```python
from build123d import *

# Parameters (mm, degrees)
SKETCH1_W           = 10
SKETCH1_H           = 10
SKETCH1_R           = 1.5
BOSS_EXTRUDE1_DEPTH = 5
FILLET1_R           = 1.5
SKETCH2_R           = 1.6
BOSS_EXTRUDE2_DEPTH = 1
SKETCH3_R           = 2.25
CUT_EXTRUDE1_DEPTH  = 4


with BuildPart() as part:
    # Sketch1 → Boss-Extrude1 (new body)
    with BuildSketch(Plane.XY):
        with Locations((-140, 155.5)):
            Rectangle(SKETCH1_W, SKETCH1_H)
        with Locations((-140, 155.5)):
            Circle(SKETCH1_R, mode=Mode.SUBTRACT)
    extrude(amount=BOSS_EXTRUDE1_DEPTH)

    # Fillet1
    fillet1_edges = [part.edges().sort_by_distance(p)[0] for p in [
        (-145, 160.5, 2.5),
        (-135, 160.5, 2.5),
        (-135, 150.5, 2.5),
        (-145, 150.5, 2.5),
    ]]
    fillet(fillet1_edges, radius=FILLET1_R)

    # Sketch2 → Boss-Extrude2 (add)
    with BuildSketch(Plane.XY.offset(5)):
        with Locations((-140, 155.5)):
            Circle(SKETCH2_R)
    extrude(amount=-BOSS_EXTRUDE2_DEPTH)

    # Sketch3 → Cut-Extrude1 (cut)
    with BuildSketch(Plane(origin=(0, 0, 0), x_dir=(-1, 0, 0), z_dir=(0, 0, -1))):
        with Locations((140, 155.5)):
            Circle(SKETCH3_R)
    extrude(amount=-CUT_EXTRUDE1_DEPTH, mode=Mode.SUBTRACT)


solid = part.part
```
For this review, take the finished solid that the model builds, in its own axes (mm). A direction names the side the tool comes from. Round coordinates to 2 decimals unless told otherwise and drop trailing zeros. Write each loop counter-clockwise with the first axis right and the second up, starting at its lowest first coordinate (ties: lowest second). Pieces come first, ordered by that corner, then holes. Notation, with made-up numbers: (86.5, 53) - (131.5, 53) arc R19 cw to (131.5, 89) - close; hole circle Ø11 at (32, -33.5). An arc over 180 degrees is marked (long way). Answer as CSV lines item,"result". Start each with the question number.
(1) Add section A-A, the plane y = 155.5. State the section outline as (x, z) points.
(2) Mouldability with a two-part tool opening along Y and no side actions: class faces 3 (the cylindrical face through (-135.45, 150.93, 2.54)), 4 (the flat face through (-140, 158, 0)), 5 (the flat face through (-140, 156, 4)) as +Y half, -Y half, draft (parallel to the pull), parting line (faces both ways), or undercut.
(3) Add section B-B, the plane z = 1.7. State the section outline as (x, y) points, plus the area to 3 significant figures.
(4) Add section D-D, the plane y = 159.5. State the section outline as (x, z) points, plus the area to 3 significant figures.
(5) Machinability: for faces 1 (the cylindrical face through (-142.08, 154.64, 1.97)), 2 (the cylindrical face through (-144.57, 160.05, 2.54)), which of the approach directions +Z, -Z, +X, -X, +Y, -Y give a long, thin tool a straight path to every point of the face, cutting with its end or side? Answer none if there is none.
(6) For line 1 (Y direction, x = -140, z = 2.55); line 2 (X direction, y = 155.5, z = 1.35); line 3 (Z direction, x = -140.75, y = 156.5), list the stretches that pass through material, from the lowest coordinate up.
(7) For pin 1 (2.5 mm diameter, centred on x = -140, y = 155.5, fed in from -Z), flat-tipped, find the tip position at first contact; note if it passes through.
(8) Add section C-C, the plane x = -140. State the section outline as (y, z) points, plus the area to 3 significant figures.
From the geometry:
1,outline,"(-145, 0) - (-142.25, 0) - (-142.25, 4) - (-137.75, 4) - (-137.75, 0) - (-135, 0) - (-135, 5) - (-145, 5) - close"
2,face 3,"-Y half"
2,face 4,"draft"
2,face 5,"undercut"
3,outline,"(-145, 152) arc R1.5 ccw to (-143.5, 150.5) - (-136.5, 150.5) arc R1.5 ccw to (-135, 152) - (-135, 159) arc R1.5 ccw to (-136.5, 160.5) - (-143.5, 160.5) arc R1.5 ccw to (-145, 159) - close; hole circle Ø4.5 at (-140, 155.5)"
3,area,"82.2 mm²"
4,outline,"(-144.91, 0) - (-135.09, 0) - (-135.09, 5) - (-144.91, 5) - close"
4,area,"49.1 mm²"
5,face 1,"-Z"
5,face 2,"+Z, -Z, -X, +Y"
6,line 1,"y = 150.5 to 153.25, 157.75 to 160.5"
6,line 2,"x = -145 to -142.25, -137.75 to -135"
6,line 3,"z = 4 to 5"
7,pin 1,"stops at z = 4"
8,outline,"(150.5, 0) - (153.25, 0) - (153.25, 4) - (157.75, 4) - (157.75, 0) - (160.5, 0) - (160.5, 5) - (150.5, 5) - close"
8,area,"32.0 mm²"
